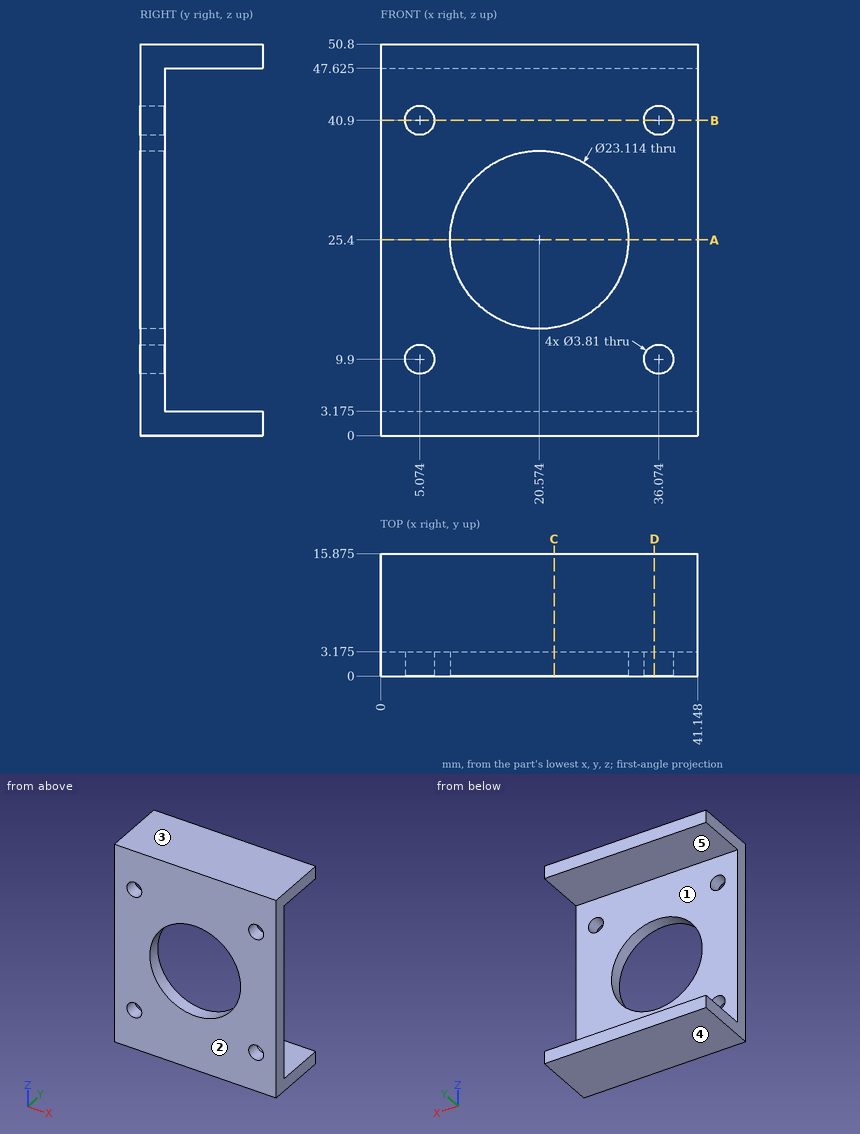
Study the drawing (mm; zero at the part's minimum x, y, z) and answer. A direction names the side the tool comes from. Give positions to 0.01 mm unless a question says otherwise; leave off trailing zeros. Loops run counter-clockwise (first coordinate to the right, second up) from the corner with the lowest first, then second, coordinate; pieces in that order, holes last. Notation, with made-up numbers: (-4, -26.5) - (39, -26.5) arc R15 ccw to (39, -2.5) - close; hole circle Ø6 at (62.5, 45.25). An arc over 180 degrees is marked (long way). Return JSON: item names as keys, results as strings. Group by question number.
1. Find section C-C (x = 22.5). Write down the section's boundary in (y, z) (3 decimals).
2. Find section B-B (z = 40.9). Write down the section's boundary in (x, y) (3 decimals).
3. Determine the mould class of the marked faces 1, 2 and 3 for opening direction Z: pulls with the +Z half, pulls with the -Z half, needs draft (parallel to the pull), parting line crosses it, or undercut.
4. Given pin 1 Ø2.5 at (x, z) = (36.074, 9.9) entering from -Y; pin 2 Ø6 at (x, z) = (5.074, 40.9) entering from +Y (3 decimals), each flat-ended and moving along its own axis, determine where each tip first touches the part or whether it passes through.
5. Which of the six approach directions +Z, -Z, +X, -X, +Y, -Y give full straight-line access (tool end or side, diameter ignored) to the marked faces 4 and 5?
6. Straight lines are drawn through the part: line 1 (X direction, y = 0.75, z = 40.9); line 2 (Z direction, x = 16.5, y = 8) (3 decimals); line 3 (Y direction, x = 38, z = 25) (3 decimals). For each, find the intervals that lie inside material, in ascending order. Write a range as [from, to].
7. Find section D-D (x = 35.5). Write down the section's boundary in (y, z) (3 decimals), then the cut area to 3 significant figures.
8. Find section A-A (z = 25.4). Write down the section's boundary in (x, y) (3 decimals).
Verdict:
{
 "1": {"outline": "(0, 0) - (15.875, 0) - (15.875, 3.175) - (3.175, 3.175) - (3.175, 14.005) - (0, 14.005) - close; (0, 36.795) - (3.175, 36.795) - (3.175, 47.625) - (15.875, 47.625) - (15.875, 50.8) - (0, 50.8) - close"},
 "2": {"outline": "(0, 0) - (3.169, 0) - (3.169, 3.175) - (0, 3.175) - close; (6.979, 0) - (34.169, 0) - (34.169, 3.175) - (6.979, 3.175) - close; (37.979, 0) - (41.148, 0) - (41.148, 3.175) - (37.979, 3.175) - close"},
 "3": {"face 1": "undercut", "face 2": "needs draft", "face 3": "pulls with the +Z half"},
 "4": {"pin 1": "passes through", "pin 2": "stops at y = 3.175"},
 "5": {"face 4": "-Z, +X, -X, +Y, -Y", "face 5": "+X, -X, +Y"},
 "6": {"line 1": "x = [0, 3.17], [6.98, 34.17], [37.98, 41.15]", "line 2": "z = [0, 3.175], [47.625, 50.8]", "line 3": "y = [0, 3.175]"},
 "7": {"outline": "(0, 0) - (15.875, 0) - (15.875, 3.175) - (3.175, 3.175) - (3.175, 8.084) - (0, 8.084) - close; (0, 11.716) - (3.175, 11.716) - (3.175, 39.084) - (0, 39.084) - close; (0, 42.716) - (3.175, 42.716) - (3.175, 47.625) - (15.875, 47.625) - (15.875, 50.8) - (0, 50.8) - close", "area": "219 mm^2"},
 "8": {"outline": "(0, 0) - (9.017, 0) - (9.017, 3.175) - (0, 3.175) - close; (32.131, 0) - (41.148, 0) - (41.148, 3.175) - (32.131, 3.175) - close"}
}
